The figure shows three views and two pictorial views of one solid part (mm, origin at its lowest corner). Answer the questions. Give positions to 0.01 mm unless a question says otherwise; leave off trailing zeros. Write each loop counter-clockwise with the first axis right and the second up, starting at its lowest first coordinate (ties: lowest second). Pieces come first, ordered by that corner, then holes. Notation, with made-up numbers: (45, -8) - (61, -8) arc R9 cw to (61, 4) - close; hole circle Ø5 at (86.25, 29.25). An arc over 180 degrees is marked (long way). Write each question's results on one line, items separated by ' | '. Start each with the question number.
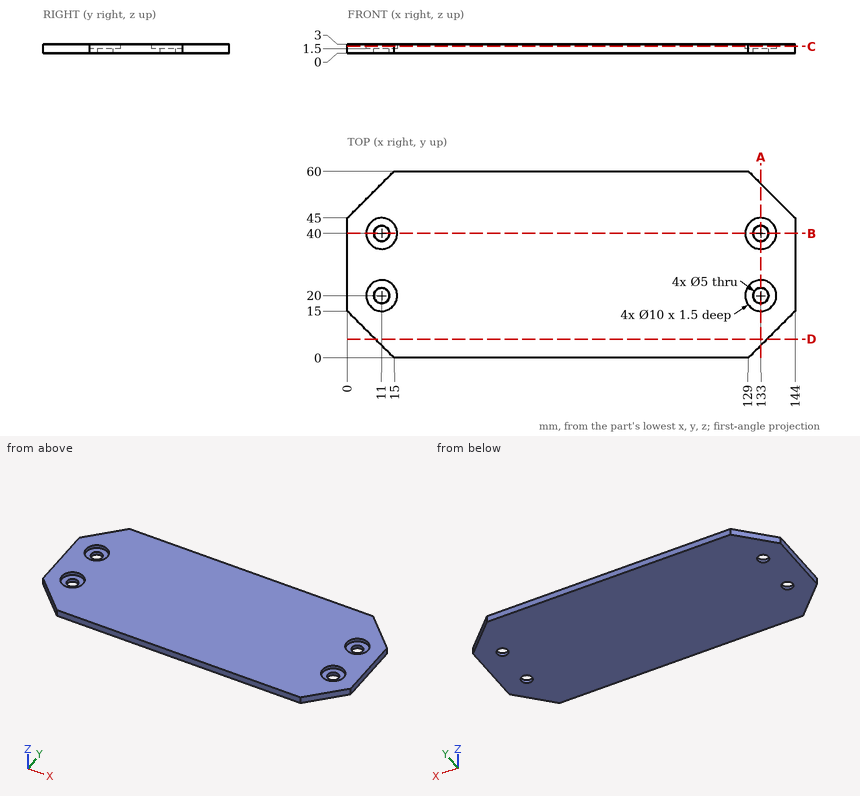
Q1. Consider L1, parallel to X at y = 19.5, z = 2.65; L2, parallel to X at y = 40, z = 0.4; L3, parallel to Y at x = 133, z = 2.5. Determine where each line is inside the solid, lowest interval first.
Q2. A cutting plane is placed at B-B, the plane y = 40. Write down the section's boundary in (x, z), and give its area (3 significant figures).
Q3. A cutting plane is placed at D-D, the plane y = 6. Write down the section's boundary in (x, z).
Q4. A cutting plane is placed at C-C, the plane z = 2.2. Write down the section's boundary in (x, y), and give its area (3 significant figures).
Q5. A cutting plane is placed at A-A, the plane x = 133. Write down the section's boundary in (y, z).
Q6. Given pin 1 (4.5 mm diameter, centred on x = 11, y = 40, fed in from +Z); pin 2 (1.5 mm diameter, centred on x = 109, y = 40.5, fed in from -Z); pin 3 (8 mm diameter, centred on x = 11, y = 20, fed in from +Z), each flat-ended and moving along its own axis, determine where each tip first touches the part or whether it passes through.
Result:
1) L1: x = 0 to 6.03, 15.97 to 128.03, 137.97 to 144 | L2: x = 0 to 8.5, 13.5 to 130.5, 135.5 to 144 | L3: y = 4 to 15, 25 to 35, 45 to 56
2) outline: (0, 0) - (8.5, 0) - (8.5, 1.5) - (6, 1.5) - (6, 3) - (0, 3) - close; (13.5, 0) - (130.5, 0) - (130.5, 1.5) - (128, 1.5) - (128, 3) - (16, 3) - (16, 1.5) - (13.5, 1.5) - close; (135.5, 0) - (144, 0) - (144, 3) - (138, 3) - (138, 1.5) - (135.5, 1.5) - close | area: 387 mm2
3) outline: (9, 0) - (135, 0) - (135, 3) - (9, 3) - close
4) outline: (0, 15) - (15, 0) - (129, 0) - (144, 15) - (144, 45) - (129, 60) - (15, 60) - (0, 45) - close; hole circle Ø10 at (11, 20); hole circle Ø10 at (11, 40); hole circle Ø10 at (133, 20); hole circle Ø10 at (133, 40) | area: 7,880 mm2
5) outline: (4, 0) - (17.5, 0) - (17.5, 1.5) - (15, 1.5) - (15, 3) - (4, 3) - close; (22.5, 0) - (37.5, 0) - (37.5, 1.5) - (35, 1.5) - (35, 3) - (25, 3) - (25, 1.5) - (22.5, 1.5) - close; (42.5, 0) - (56, 0) - (56, 3) - (45, 3) - (45, 1.5) - (42.5, 1.5) - close
6) pin 1: passes through | pin 2: stops at z = 0 | pin 3: stops at z = 1.5
